Can you work these out from the model? Positions are in its coordinate system, mm. A direction names the side the tool comes from. Give positions to 0.01 mm unless a question says otherwise; leave off trailing zeros. Write each loop counter-clockwise with the first axis right and the second up, starting at its lowest first coordinate (ties: lowest second). Pieces come first, ordered by that corner, then holes.
1. Suppose I cut it at C-C (x = 7.75). Please give me the cut outline in (y, z), and give its area (3 significant figures).
2. I'm going to push flat-ended pins straight in: pin 1 (1.5 mm diameter, centred on x = 3.5, y = 0.5, fed in from -Z); pin 2 (0.9 mm diameter, centred on x = 13, y = 1, fed in from +Z); pin 3 (1.5 mm diameter, centred on x = 13.5, y = 2, fed in from -Z). Where does each tip first touch, or does it pass through?
3. Suppose I cut it at B-B (x = 0). Please give me the cut outline in (y, z) (3 decimals), and give its area (4 significant figures).
4. Suppose I cut it at A-A (z = 0). Please give me the cut outline in (x, y) (3 decimals).
5. Thinking about a two-plate mould opening in X: for faces 5 (the flat face through (-7.7, 1.48, 11.14)), 6 (the flat face through (-3.426, 1.479, 13.1)), 7 (the cylindrical face through (-11.481, 1.479, -9.654)), 8 (the flat face through (11.82, 1.48, 2.07)), which applies, pulls with the +X half, pulls with the -X half, needs draft (parallel to the pull), parting line crosses it, or undercut?
6. On a 3-axis mill with a long thin cutter (end or side, diameter ignored), from which of +Z, -Z, +X, -X, +Y, -Y can I reach the whole of each face in a straight line? I mean faces 1 (the flat face through (-13, 1, -1.099)), 2 (the cylindrical face through (2.62, 1.48, -14.77)), 3 (the flat face through (-9.632, 1.479, -9.517)), 4 (the flat face through (-12.267, 1.479, 5.634)). Say none if no direction works.
7. If I drill on probe 1 along X at (y, z) = (1.6, 0) (3 decimals); probe 2 along Z at (x, y) = (-8, 1.75); probe 3 along X at (y, z) = (2.7, -12.5), over which ranges is the centre line in solid material (lowest first)?
```python
from build123d import *

# Parameters (mm, degrees)
SKETCH_1_R               = 15
EXTRUDE_1_DEPTH          = 3
CUT_EXTRUDE_START        = -3
CUT_EXTRUDE_1_DEPTH      = 3
PATTERN_CIRCULAR_1_COUNT = 18
SKETCH_3_R               = 2.375
CUT_EXTRUDE_2_DEPTH      = 10


with BuildPart() as part:
    # Эскиз1 → Бобышка-Вытянуть1 (new body)
    with BuildSketch(Plane(origin=(0, 0, 0), x_dir=(1, 0, 0), z_dir=(0, 1, 0))):
        with Locations(Location((0, 0, 0), (0, 0, 270))):
            Circle(SKETCH_1_R)
    extrude(amount=EXTRUDE_1_DEPTH)

    # Эскиз2 → Вырез-Вытянуть1 (cut)
    with BuildSketch(Plane(origin=(0, 3, 0), x_dir=(1, 0, 0), z_dir=(0, 1, 0)).offset(CUT_EXTRUDE_START)):
        with BuildLine():
            ThreePointArc((1.515448005, 14.923250897), (0.75869511, 14.980800437), (0, 15))
            Line((0, 15), (0, 12))
            Line((0, 12), (1, 12))
            Line((1, 12), (1.515448005, 14.923250897))
        make_face()
        with BuildLine():
            Line((0, 12), (0, 15))
            ThreePointArc((0, 15), (-0.75869511, 14.980800437), (-1.515448005, 14.923250897))
            Line((-1.515448005, 14.923250897), (-1, 12))
            Line((-1, 12), (0, 12))
        make_face()
    cut_extrude_1 = extrude(amount=CUT_EXTRUDE_1_DEPTH, mode=Mode.SUBTRACT)

    # Круговой массив1: Вырез-Вытянуть1 ×18 about axis
    pattern_circular_1_axis = Axis((0, 0, 0), (0, 1, 0))
    for i in range(1, PATTERN_CIRCULAR_1_COUNT):
        add(cut_extrude_1.rotate(pattern_circular_1_axis, i * 360 / PATTERN_CIRCULAR_1_COUNT), mode=Mode.SUBTRACT)

    # Эскиз3 → Вырез-Вытянуть2 (cut)
    with BuildSketch(Plane(origin=(0, 3, 0), x_dir=(1, 0, 0), z_dir=(0, 1, 0))):
        with Locations(Location((0, 0, 0), (0, 0, 270))):
            Circle(SKETCH_3_R)
    extrude(amount=-CUT_EXTRUDE_2_DEPTH, mode=Mode.SUBTRACT)


solid = part.part
```
Checks:
1. outline: (0, -12.84) - (3, -12.84) - (3, -11.23) - (0, -11.23) - close; (0, -9.16) - (3, -9.16) - (3, 9.16) - (0, 9.16) - close; (0, 11.23) - (3, 11.23) - (3, 12.84) - (0, 12.84) - close
1. area: 64.7 mm2
2. pin 1: stops at z = -14.75
2. pin 2: stops at z = 6.06
2. pin 3: stops at z = -6.15
3. outline: (0, -12) - (3, -12) - (3, -2.375) - (0, -2.375) - close; (0, 2.375) - (3, 2.375) - (3, 12) - (0, 12) - close
3. area: 57.75 mm2
4. outline: (-15, 0) - (-2.375, 0) - (-2.375, 3) - (-15, 3) - close; (2.375, 0) - (15, 0) - (15, 3) - (2.375, 3) - close
5. face 5: undercut
5. face 6: undercut
5. face 7: pulls with the -X half
5. face 8: pulls with the +X half
6. face 1: -X, +Y, -Y
6. face 2: -Z, +X, +Y, -Y
6. face 3: -Z, +Y, -Y
6. face 4: +Y, -Y
7. probe 1: x = -15 to -2.375, 2.375 to 15
7. probe 2: z = -12.69 to -11.66, -8.95 to 8.95, 11.66 to 12.69
7. probe 3: x = -8.29 to -5.95, -3.32 to -1.09, 1.09 to 3.32, 5.95 to 8.29
